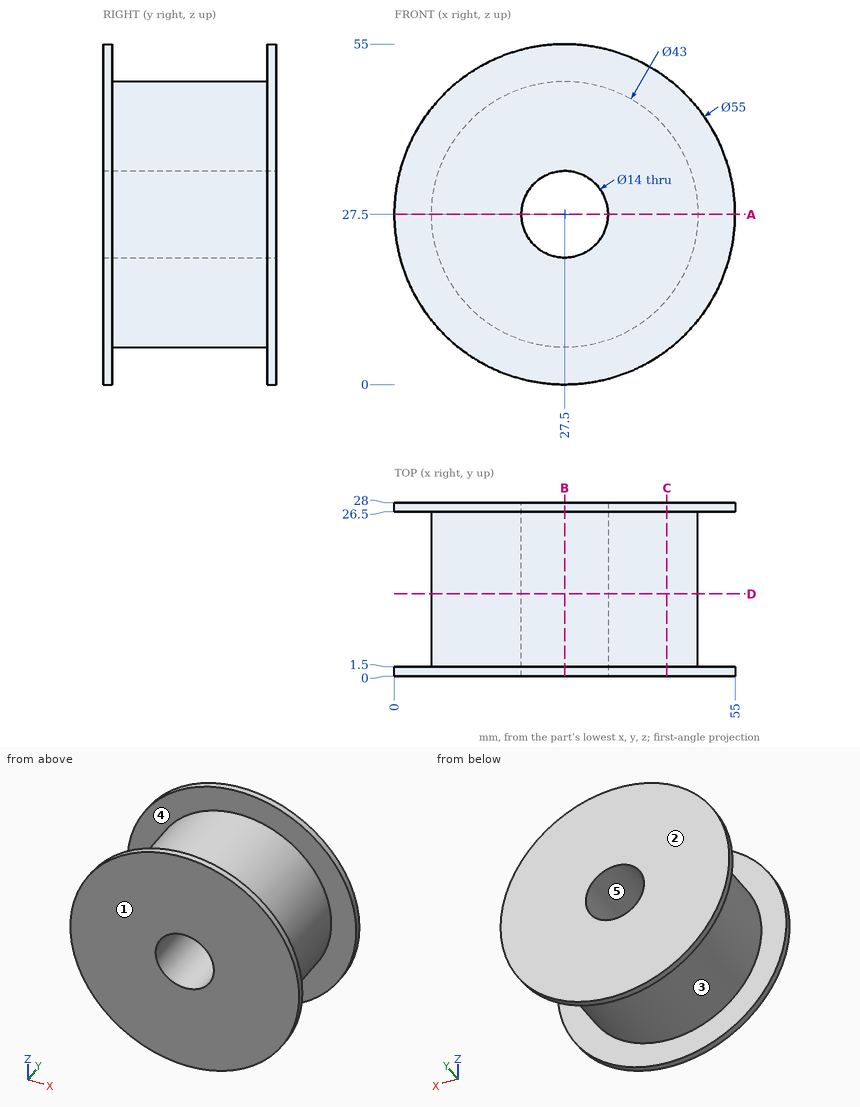
Geometry check sheet. Reference: drawing and pictorial views, mm from the part's lowest x, y, z. A direction names the side the tool comes from. Round coordinates to 2 decimals unless told otherwise and drop trailing zeros. Loops run counter-clockwise (first coordinate to the right, second up) from the corner with the lowest first, then second, coordinate; pieces in that order, holes last. Notation, with made-up numbers: M 87.5,18.5 L 121.5,18.5 A7 ccw 121.5,22.5 Z; hole C -9.75,76.5 d5. An arc over 180 degrees is marked long. Return JSON: item names as keys, results as strings. Group by question number.
(1) Section check C-C, the plane x = 44. Enter the section's corners in (y, z).
(2) Section check B-B, the plane x = 27.5. Enter the section's corners in (y, z), and give its area (3 significant figures).
(3) Set-up check for the marked faces 4 and 5: record each of +Z, -Z, +X, -X, +Y, -Y from which the full face is reachable in a straight line by a thin tool's end or side.
(4) Section check A-A, the plane z = 27.5. Enter the section's corners in (x, y).
(5) Scan lines: line 1 along X through (y, z) = (21.5, 27.5); line 2 along Y through (x, z) = (9.5, 41); line 3 along X through (y, z) = (18, 28.5). Record each from-to range of solid material in increasing order. Write a range as [from, to].
(6) Section check D-D, the plane y = 13.25. Enter the section's corners in (x, z), and give its area (3 significant figures).
(7) Go/stop test with flat-tipped pins: pin 1 (1 mm diameter, centred on y = 12.5, z = 23, fed in from -X); pin 2 (8 mm diameter, centred on x = 14.5, y = 21, fed in from -Z); pin 3 (6 mm diameter, centred on y = 22.5, z = 25.5, fed in from +X). Record where each tip stops, or that it passes through.
(8) Mould release check, pull along Y, two halves, no side actions. Record for the marked faces 1, 2 and 3: pulls with the +Y half, pulls with the -Y half, needs draft (parallel to the pull), parting line crosses it, or undercut.
Data:
{
 "1": {"outline": "M 0,5.5 L 1.5,5.5 L 1.5,13.72 L 26.5,13.72 L 26.5,5.5 L 28,5.5 L 28,49.5 L 26.5,49.5 L 26.5,41.28 L 1.5,41.28 L 1.5,49.5 L 0,49.5 Z"},
 "2": {"outline": "M 0,0 L 1.5,0 L 1.5,6 L 26.5,6 L 26.5,0 L 28,0 L 28,20.5 L 0,20.5 Z; M 0,34.5 L 28,34.5 L 28,55 L 26.5,55 L 26.5,49 L 1.5,49 L 1.5,55 L 0,55 Z", "area": "848 mm²"},
 "3": {"face 4": "none", "face 5": "+Y, -Y"},
 "4": {"outline": "M 0,0 L 20.5,0 L 20.5,28 L 0,28 L 0,26.5 L 6,26.5 L 6,1.5 L 0,1.5 Z; M 34.5,0 L 55,0 L 55,1.5 L 49,1.5 L 49,26.5 L 55,26.5 L 55,28 L 34.5,28 Z"},
 "5": {"line 1": "[6, 20.5], [34.5, 49]", "line 2": "[0, 1.5], [26.5, 28]", "line 3": "[6.02, 20.57], [34.43, 48.98]"},
 "6": {"outline": "C 27.5,27.5 d43; hole C 27.5,27.5 d14", "area": "1,300 mm²"},
 "7": {"pin 1": "x = 6.38", "pin 2": "z = 7.97", "pin 3": "x = 49"},
 "8": {"face 1": "pulls with the -Y half", "face 2": "pulls with the +Y half", "face 3": "undercut"}
}
